Part model, mm, in its own coordinate system. A direction names the side the tool comes from. Coordinates: 2 decimals unless noted, no trailing zeros. Loops run counter-clockwise (first coordinate to the right, second up) from the corner with the lowest first, then second, coordinate; pieces in that order, holes last.
```python
from build123d import *

# Parameters (mm, degrees)
F0_R     = 50
F1_DEPTH = 3.17
F2_R     = 2.5
F3_DEPTH = 25
F5_DEPTH = 25


with BuildPart() as f1:
    # F0 (on Front) → F1 (new body)
    with BuildSketch(Plane.XZ):
        Circle(F0_R)
    extrude(amount=F1_DEPTH)

    # F2 (on face) → F3 (cut)
    with BuildSketch(Plane.XZ.offset(3.17)):
        Circle(F2_R)
    extrude(amount=-F3_DEPTH, mode=Mode.SUBTRACT)

    # F4 (on face) → F5 (cut)
    with BuildSketch(Plane.XZ.offset(3.17)):
        with BuildLine():
            Line((-22.7931910082, 31.3721360136), (-15.0621287485, 47.6773769996))
            ThreePointArc((-15.0621287485, 47.6773769996), (-20.5685569707, 45.5733964517), (-25.7891029355, 42.8359915233))
            Line((-25.7891029355, 42.8359915233), (-22.7931910082, 31.3721360136))
        make_face()
        with BuildLine():
            Line((0, 38.7780927122), (15.8385409393, 47.4251053864))
            ThreePointArc((15.8385409393, 47.4251053864), (10.1470581921, 48.9595466691), (4.3145415402, 49.8134994886))
            Line((4.3145415402, 49.8134994886), (0, 38.7780927122))
        make_face()
        with BuildLine():
            ThreePointArc((40.6894263206, 29.0580554357), (36.9868420114, 33.6448141327), (32.7701777935, 37.7639437478))
            Line((32.7701777935, 37.7639437478), (22.7931910082, 31.3721360136))
            Line((22.7931910082, 31.3721360136), (40.6894263206, 29.0580554357))
        make_face()
        with BuildLine():
            ThreePointArc((50, 0), (49.6761310759, 5.6817252069), (48.7087199469, 11.2898450446))
            Line((48.7087199469, 11.2898450446), (36.8801577634, 11.9830896575))
            Line((36.8801577634, 11.9830896575), (49.9983338301, -0.4081840445))
            ThreePointArc((49.9983338301, -0.4081840445), (49.9995834558, -0.2040937225), (50, 0))
        make_face()
        with BuildLine():
            ThreePointArc((40.2095771974, -29.7185110934), (43.4276824703, -24.7797577725), (46.0421866292, -19.4965907379))
            Line((46.0421866292, -19.4965907379), (36.8801577634, -11.9830896575))
            Line((36.8801577634, -11.9830896575), (40.2095771974, -29.7185110934))
        make_face()
        with BuildLine():
            ThreePointArc((15.0621287485, -47.6773769996), (20.5685569707, -45.5733964517), (25.7891029355, -42.8359915233))
            Line((25.7891029355, -42.8359915233), (22.7931910082, -31.3721360136))
            Line((22.7931910082, -31.3721360136), (15.0621287485, -47.6773769996))
        make_face()
        with BuildLine():
            ThreePointArc((-15.8385409393, -47.4251053864), (-10.1470581921, -48.9595466691), (-4.3145415402, -49.8134994886))
            Line((-4.3145415402, -49.8134994886), (0, -38.7780927122))
            Line((0, -38.7780927122), (-15.8385409393, -47.4251053864))
        make_face()
        with BuildLine():
            Line((-22.7931910082, -31.3721360136), (-40.6894263206, -29.0580554357))
            ThreePointArc((-40.6894263206, -29.0580554357), (-36.9868420114, -33.6448141327), (-32.7701777935, -37.7639437478))
            Line((-32.7701777935, -37.7639437478), (-22.7931910082, -31.3721360136))
        make_face()
        with BuildLine():
            Line((-36.8801577634, -11.9830896575), (-49.9983338301, 0.4081840445))
            ThreePointArc((-49.9983338301, 0.4081840445), (-49.6989093188, -5.4789061428), (-48.7087199469, -11.2898450446))
            Line((-48.7087199469, -11.2898450446), (-36.8801577634, -11.9830896575))
        make_face()
        with BuildLine():
            Line((-36.8801577634, 11.9830896575), (-40.2095771974, 29.7185110934))
            ThreePointArc((-40.2095771974, 29.7185110934), (-43.4276824703, 24.7797577725), (-46.0421866292, 19.4965907379))
            Line((-46.0421866292, 19.4965907379), (-36.8801577634, 11.9830896575))
        make_face()
    extrude(amount=-F5_DEPTH, mode=Mode.SUBTRACT)


solid = f1.part
```
Q1. Saw through at D-D (x = -19.5). List the corners of the cut face in (y, z).
Q2. Probe line 1 (X direction, y = -1, z = 41.5); line 2 (Z direction, x = 45, y = -0.05); line 3 (X direction, y = -1.1, z = 12.5). List the from-to ranges inside material, lowest first.
Q3. Drop flat-ended pins along their axis: P1, Ø1, axis at x = -17, y = -1.5, coming from the +Z side; P2, Ø1.5, axis at x = -0.5, y = -1, coming from the -Z side; P3, Ø3, axis at x = 0, z = 0, coming from the -Y side. Give the stop position or say it passes through.
Q4. Saw through at B-B (x = 28). List the corners of the cut face in (y, z).
Q5. Tool access for faces 1 (the cylindrical face through (5.342, -1.563, -49.714)), 2 (the flat face through (38.522, -1.607, -20.727)), 3 (the flat face through (-27.85, -1.61, -34.61)): list every direction of +Z, -Z, +X, -X, +Y, -Y with a clear straight run to the whole face (end or side of a thin tool).
Q6. Mould opens along X. For faces 4 (the cylindrical face through (-0.54, -1.61, -2.44)), 5 (the cylindrical face through (33.54, -1.56, -37.08)), 6 (the cylindrical face through (-24.9, -1.56, -43.36)) say: released by +X, released by -X, zero draft, split by the parting line, or undercut.
Q7. Saw through at C-C (z = 16.5). List the corners of the cut face in (x, y).
Checked values:
1. outline: (-3.17, -46.04) - (0, -46.04) - (0, 38.32) - (-3.17, 38.32) - close
2. line 1: x = -27.89 to -25.44, -17.99 to 1.06, 4.99 to 27.89
2. line 2: z = -18.64 to 4.31, 11.51 to 21.79
2. line 3: x = -48.41 to -37.51, -36.98 to 48.41
3. P1: stops at z = 44.64
3. P2: stops at z = -50
3. P3: passes through
4. outline: (-3.17, -41.42) - (0, -41.42) - (0, 30.7) - (-3.17, 30.7) - close; (-3.17, 34.71) - (0, 34.71) - (0, 41.42) - (-3.17, 41.42) - close
5. face 1: -Z, +Y, -Y
5. face 2: +Y, -Y
5. face 3: -X, +Y, -Y
6. face 4: undercut
6. face 5: released by +X
6. face 6: released by -X
7. outline: (-47.2, -3.17) - (-42.39, -3.17) - (-42.39, 0) - (-47.2, 0) - close; (-37.73, -3.17) - (47.2, -3.17) - (47.2, 0) - (-37.73, 0) - close
